Here's how the part is built. I have some questions about the finished solid (model axes, mm). A direction names the side the tool comes from. Round coordinates to 2 decimals unless told otherwise and drop trailing zeros. Loops run counter-clockwise (first coordinate to the right, second up) from the corner with the lowest first, then second, coordinate; pieces in that order, holes last. Notation, with made-up numbers: M -13,18 L 45,18 A28 cw 45,47 Z; hole C 60,56 d6. An arc over 180 degrees is marked long. Write item = value, one per line. Start each with the question number.
from build123d import *

# Parameters (mm, degrees)
ESQUISSE1_R        = 22.5
ESQUISSE1_R_2      = 1.5
BOSS_EXTRU_1_DEPTH = 3
ESQUISSE2_R        = 15
BOSS_EXTRU_2_DEPTH = 100
CONG_1_R           = 10


with BuildPart() as part:
    # Esquisse1 → Boss.-Extru.1 (new body)
    with BuildSketch(Plane.XY):
        Circle(ESQUISSE1_R)
        with Locations((0, 19)):
            Circle(ESQUISSE1_R_2, mode=Mode.SUBTRACT)
        with Locations((19, 0)):
            Circle(ESQUISSE1_R_2, mode=Mode.SUBTRACT)
        with Locations((0, -19)):
            Circle(ESQUISSE1_R_2, mode=Mode.SUBTRACT)
        with Locations((-19, 0)):
            Circle(ESQUISSE1_R_2, mode=Mode.SUBTRACT)
    extrude(amount=BOSS_EXTRU_1_DEPTH)

    # Esquisse2 → Boss.-Extru.2 (add)
    with BuildSketch(Plane(origin=(0, 0, 0), x_dir=(-1, 0, 0), z_dir=(0, 0, -1))):
        Circle(ESQUISSE2_R)
    extrude(amount=BOSS_EXTRU_2_DEPTH)

    # Congé1
    cong_1_edges = [part.edges().sort_by_distance(p)[0] for p in [
        (15, 0, -100),
    ]]
    fillet(cong_1_edges, radius=CONG_1_R)


solid = part.part
Item 1: I want a section at A-A, the plane y = 0. State how many separate pieces and enclosed holes the cut face has, then the cut area to 3 significant figures.
Item 2: We'd pull the mould along X, two halves only. Please class faces 1 (the flat face through (0, 0, 3)), 2 (the cylindrical face through (10.382, -19.961, 1.479)), 3 (the cylindrical face through (-20.5, 0.07, 1.48)): released by +X, released by -X, zero draft, split by the parting line, or undercut.
Item 3: For faces 4 (the cylindrical face through (-0.195, -17.513, 1.479)), 5 (the cylindrical face through (14.985, 0.66, -44.37)), which set-ups out of +Z, -Z, +X, -X, +Y, -Y let a thin tool reach every point of the face, with its end or its side?
Item 4: Will these pins go through, and if not, where does the flat tip stop? pin 1 Ø12 at (x, z) = (-18, -83.5) entering from +Y; pin 2 Ø10 at (y, z) = (10, -14) entering from +X; pin 3 Ø2 at (y, z) = (6, -20.5) entering from -X.
Item 5: I want a section at B-B, the plane x = 19. List the corners of the cut face in (y, z) for me, then the cut area to 3 significant figures.
Item 6: Please list where these lines run through material, in increasing order: line 1 (Z direction, x = -10.5, y = -16); line 2 (Y direction, x = -19, z = 1.25); line 3 (Y direction, x = -9.5, z = -30). Write a range as [from, to].
Worked out:
q1.separate_pieces = 3
q1.enclosed_holes = 0
q1.area = 3,070 mm2
q2.face_1 = zero draft
q2.face_2 = split by the parting line
q2.face_3 = undercut
q3.face_4 = +Z, -Z
q3.face_5 = -Z
q4.pin_1 = 9
q4.pin_2 = 14.14
q4.pin_3 = -14.14
q5.outline = M -12.05,0 L -1.5,0 L -1.5,3 L -12.05,3 Z; M 1.5,0 L 12.05,0 L 12.05,3 L 1.5,3 Z
q5.area = 63.3 mm2
q6.line_1 = [0, 3]
q6.line_2 = [-12.05, -1.5], [1.5, 12.05]
q6.line_3 = [-11.61, 11.61]
